Work out the finished part from the listing and answer in its coordinate system (mm). Face numbers are marked on the shaded views. A direction names the side the tool comes from. Give positions to 0.01 mm unless a question says otherwise; leave off trailing zeros. Loops run counter-clockwise (first coordinate to the right, second up) from the corner with the lowest first, then second, coordinate; pieces in that order, holes last. Notation, with made-up numbers: (-2, -21.75) - (30, -21.75) arc R24 ccw to (30, 17.25) - close; hole circle Ø11 at (-32, -8). An arc over 180 degrees is marked (long way). Use CSV: the item, a comma, the result in double quotes.
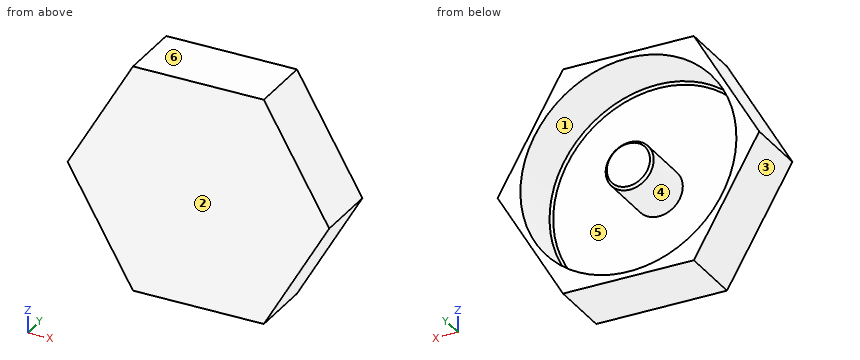
from build123d import *

# Parameters (mm, degrees)
SKETCH1_R             = 22.5
BOSS_EXTRUDE1_DEPTH   = 12
SKETCH1_R_2           = 5
BOSS_EXTRUDE1_2_DEPTH = 12
BOSS_EXTRUDE2_DEPTH   = 1.1
CHAMFER1_SIZE         = 0.5


with BuildPart() as part:
    # Sketch1 → Boss-Extrude1 (new body)
    with BuildSketch(Plane(origin=(0, 0, 0), x_dir=(1, 0, 0), z_dir=(0, 1, 0))):
        Polygon((13.625466353, -23.6), (27.250932706, 0), (13.625466353, 23.6), (-13.625466353, 23.6), (-27.250932706, 0), (-13.625466353, -23.6), align=None)
        with Locations(Location((0, 0, 0), (0, 0, 270))):
            Circle(SKETCH1_R, mode=Mode.SUBTRACT)
    extrude(amount=BOSS_EXTRUDE1_DEPTH)



with BuildPart() as body_2:
    # Sketch1 → Boss-Extrude1 2 (new body)
    with BuildSketch(Plane(origin=(0, 0, 0), x_dir=(1, 0, 0), z_dir=(0, 1, 0))):
        with Locations(Location((0, 0, 0), (0, 0, 270))):
            Circle(SKETCH1_R_2)
    extrude(amount=BOSS_EXTRUDE1_2_DEPTH)


with BuildPart() as part_1:
    add(part.part)

    add(body_2.part)  # Boss-Extrude2 merges body 2
    # Sketch2 → Boss-Extrude2 (add)
    with BuildSketch(Plane.XZ):
        Polygon((-13.625466353, -23.6), (-27.250932706, 0), (-13.625466353, 23.6), (13.625466353, 23.6), (27.250932706, 0), (13.625466353, -23.6), align=None)
    extrude(amount=BOSS_EXTRUDE2_DEPTH)

    # Chamfer1
    chamfer1_edges = [part_1.edges().sort_by_distance(p)[0] for p in [
        (0, 0, -22.5),
        (0, 12, -5),
    ]]
    chamfer(chamfer1_edges, length=CHAMFER1_SIZE)


solid = part_1.part
Item 1: Find the intervals of material crossed by line 1 (X direction, y = 9, z = 0); line 2 (X direction, y = 5.5, z = 4); line 3 (Y direction, x = 9, z = 11), in increasing order.
Determined:
line 1,"x = -27.25 to -22.5, -5 to 5, 22.5 to 27.25"
line 2,"x = -24.94 to -22.14, -3 to 3, 22.14 to 24.94"
line 3,"y = -1.1 to 0"
Item 2: Given P1, Ø4, axis at y = 3.5, z = 8.5, coming from the +X side; P2, Ø3, axis at y = 0.5, z = 13.5, coming from the +X side; P3, Ø1.5, axis at x = 12, z = 4.5, coming from the +Y side, each flat-ended and moving along its own axis, determine where each tip first touches the part or whether it passes through.
Determined:
P1,"stops at x = 23.5"
P2,"stops at x = 20.32"
P3,"stops at y = 0"
Item 3: A cutting plane is placed at A-A on y = 8. Determine the outline of the cut face in (x, z), and give its area (3 significant figures).
Determined:
outline,"(-27.25, 0) - (-13.63, -23.6) - (13.63, -23.6) - (27.25, 0) - (13.63, 23.6) - (-13.63, 23.6) - close; circle Ø10 at (0, 0); hole circle Ø45 at (0, 0)"
area,"417 mm²"
Item 4: For the marked faces 5 and 6, determine the directions among +Z, -Z, +X, -X, +Y, -Y from which every point of the face is accessible in a straight line to the end or side of a thin tool.
Determined:
face 5,"+Y"
face 6,"+Z, +X, -X, +Y, -Y"
Item 5: A cutting plane is placed at B-B on x = 0. Determine the outline of the cut face in (y, z).
Determined:
outline,"(-1.1, -23.6) - (12, -23.6) - (12, -22.5) - (0.5, -22.5) - (0, -22) - (0, -5) - (11.5, -5) - (12, -4.5) - (12, 4.5) - (11.5, 5) - (0, 5) - (0, 22) - (0.5, 22.5) - (12, 22.5) - (12, 23.6) - (-1.1, 23.6) - close"
Item 6: The mould has two halves that part along Z. Classify the marked faces 1, 2, 3 and 4: pulls with the +Z half, pulls with the -Z half, needs draft (parallel to the pull), parting line crosses it, or undercut.
Determined:
face 1,"undercut"
face 2,"needs draft"
face 3,"pulls with the -Z half"
face 4,"undercut"
